Input: part model. Units: mm. Frame: model coordinates. A direction names the side the tool comes from. Give positions to 0.01 mm unless a question says otherwise; leave off trailing zeros. Write each loop counter-clockwise with the first axis right and the second up, starting at its lowest first coordinate (ties: lowest second). Pieces come first, ordered by that corner, then holes. Notation, with made-up numbers: (54.5, 60) -> (60.5, 60) arc R23 cw to (60.5, 98) -> close; hole circle Ø1 at (-15, -33.5). An arc over 180 degrees is marked (long way). Return JSON: item names as keys, results as strings. Group by question number.
Item 1: Line query: line 1 (Z direction, x = -101, y = -100); line 2 (X direction, y = -39, z = 58); line 3 (Z direction, x = -7.5, y = -58). Output: solid intervals per line, ascending. Write a range as [from, to].
Item 2: Pin query (flat end, axial travel): P1, Ø11, axis at y = -100, z = 127.87, coming from the +X side; P2, Ø1, axis at x = -20.5, y = -170, coming from the +Z side; P3, Ø2, axis at x = -28.5, y = -69.5, coming from the -Z side; P4, Ø4, axis at y = -74, z = 99.5, coming from the +X side. Return the tip coordinate at first contact, or that it passes through.
Item 3: Section D-D, the plane y = -74.5. Return loops of the section in (x, z).
Item 4: Mould query, pull axis Y, two halves, no side actions, for faces 3 (the face through (-107.318, -93.956, 128.135)), 4 (the face through (-33, 0, 25)), 5 (the face through (-33, -200, 25)). Classes: released by +Y, released by -Y, zero draft, split by the parting line, or undercut.
Item 5: Set-up query: faces 1 (the face through (41, -99, 40)), 2 (the face through (-106.758, -102.199, 299.845)). Return all of +Z, -Z, +X, -X, +Y, -Y with unobstructed straight access to the full face (end or side cutting, diameter ignored); none if empty.
Item 6: Section A-A, the plane y = -100. Return loops of the section in (x, z).
Item 7: Section C-C, the plane x = -101.5. Return loops of the section in (y, z), then the cut area to 3 significant figures.
Item 8: Section B-B, the plane z = 240.5. Return loops of the section in (x, y).
from build123d import *

# Parameters (mm, degrees)
F0_W     = 300
F0_H     = 40
F1_DEPTH = 200
F2_W     = 40
F2_H     = 200
F3_DEPTH = 260
F5_DEPTH = 40.001
F6_R     = 50
F7_DEPTH = 40.001
F8_D     = 12.1


with BuildPart() as f1:
    # F0 (on Front) → F1 (new body)
    with BuildSketch(Plane.XZ):
        with Locations((22.9622232423, 20)):
            Rectangle(F0_W, F0_H)
    extrude(amount=F1_DEPTH)

    # F2 (on face) → F3 (join)
    with BuildSketch(Plane.XY.offset(40)):
        with Locations((-107.0377767577, -100)):
            Rectangle(F2_W, F2_H)
    extrude(amount=F3_DEPTH)

    # F4 (on face) → F5 (cut, through all)
    with BuildSketch(Plane.YZ.offset(-87.0377767577)):
        with BuildLine():
            ThreePointArc((-200, 199.8689621687), (-100, 299.8689621687), (0, 199.8689621687))
            Line((0, 199.8689621687), (0, 300))
            Line((0, 300), (-200, 300))
            Line((-200, 300), (-200, 199.8689621687))
        make_face()
    extrude(amount=-F5_DEPTH, mode=Mode.SUBTRACT)

    # F6 (on face) → F7 (cut, through all)
    with BuildSketch(Plane.YZ.offset(-87.0377767577)):
        with Locations((-100, 199.8689621687)):
            Circle(F6_R)
    extrude(amount=-F7_DEPTH, mode=Mode.SUBTRACT)

    # F8 (through all)
    with Locations(Plane.YZ.offset(-87.0377767577)):
        with Locations((-100, 271.8689621687), (-172, 199.8689621687), (-100, 127.8689621687), (-28, 199.8689621687)):
            Hole(F8_D / 2)


solid = f1.part
Answer below:
{
 "1": {"line 1": "z = [0, 121.82], [133.92, 149.87], [249.87, 265.82], [277.92, 299.87]", "line 2": "x = [-127.04, -87.04]", "line 3": "z = [0, 40]"},
 "2": {"P1": "passes through", "P2": "stops at z = 40", "P3": "stops at z = 0", "P4": "stops at x = -87.04"},
 "3": {"outline": "(-127.04, 0) -> (172.96, 0) -> (172.96, 40) -> (-87.04, 40) -> (-87.04, 156.86) -> (-127.04, 156.86) -> close; (-127.04, 242.88) -> (-87.04, 242.88) -> (-87.04, 296.56) -> (-127.04, 296.56) -> close"},
 "4": {"face 3": "undercut", "face 4": "released by +Y", "face 5": "released by -Y"},
 "5": {"face 1": "+Z, +X, +Y, -Y", "face 2": "+Z, +X, -X"},
 "6": {"outline": "(-127.04, 0) -> (172.96, 0) -> (172.96, 40) -> (-87.04, 40) -> (-87.04, 121.82) -> (-127.04, 121.82) -> close; (-127.04, 133.92) -> (-87.04, 133.92) -> (-87.04, 149.87) -> (-127.04, 149.87) -> close; (-127.04, 249.87) -> (-87.04, 249.87) -> (-87.04, 265.82) -> (-127.04, 265.82) -> close; (-127.04, 277.92) -> (-87.04, 277.92) -> (-87.04, 299.87) -> (-127.04, 299.87) -> close"},
 "7": {"outline": "(-200, 0) -> (0, 0) -> (0, 199.87) arc R100 ccw to (-200, 199.87) -> close; hole circle Ø12.1 at (-172, 199.87); hole circle Ø100 at (-100, 199.87); hole circle Ø12.1 at (-100, 127.87); hole circle Ø12.1 at (-100, 271.87); hole circle Ø12.1 at (-28, 199.87)", "area": "47,400 mm2"},
 "8": {"outline": "(-127.04, -191.37) -> (-87.04, -191.37) -> (-87.04, -129.14) -> (-127.04, -129.14) -> close; (-127.04, -70.86) -> (-87.04, -70.86) -> (-87.04, -8.63) -> (-127.04, -8.63) -> close"}
}
